Check sheet for the drawn part. Datum: minimum x, y, z corner. Units: mm. Round coordinates to 2 decimals unless told otherwise and drop trailing zeros. Write each loop counter-clockwise with the first axis right and the second up, starting at its lowest first coordinate (ties: lowest second). Pieces come first, ordered by that corner, then holes. Notation, with made-up numbers: M 63.5,24 L 75.5,24 A21 ccw 75.5,48 Z; hole C 58.25,89.25 d11. An arc over 180 degrees is marked long. One line per item, written item: value. Start each with the question number.
1. Section check B-B (y = 4.75). Record the boundary of the cut face in (x, z).
2. Section check A-A (z = 17.5). Record the boundary of the cut face in (x, y), and give its area (3 significant figures).
3. Release check for a two-part mould opening along X. For the marked faces 1, 2 and 3 record: pulls with the +X half, pulls with the -X half, needs draft (parallel to the pull), parting line crosses it, or undercut.
4. Depth check by flat-ended pin: P1, Ø1.5, axis at x = 13.5, y = 7.5, coming from the -Z side; P2, Ø3, axis at y = 12, z = 24.5, coming from the -X side; P3, Ø8, axis at y = 2, z = 10.5, coming from the -X side. Enter the tip coordinate at first touch or a pass-through.
5. Scan lines: probe 1 along Z at (x, y) = (17.5, 11); probe 2 along Z at (x, y) = (18, 6.5); probe 3 along Z at (x, y) = (10.5, 8.5). Record each from-to range of solid material in increasing order. Write a range as [from, to].
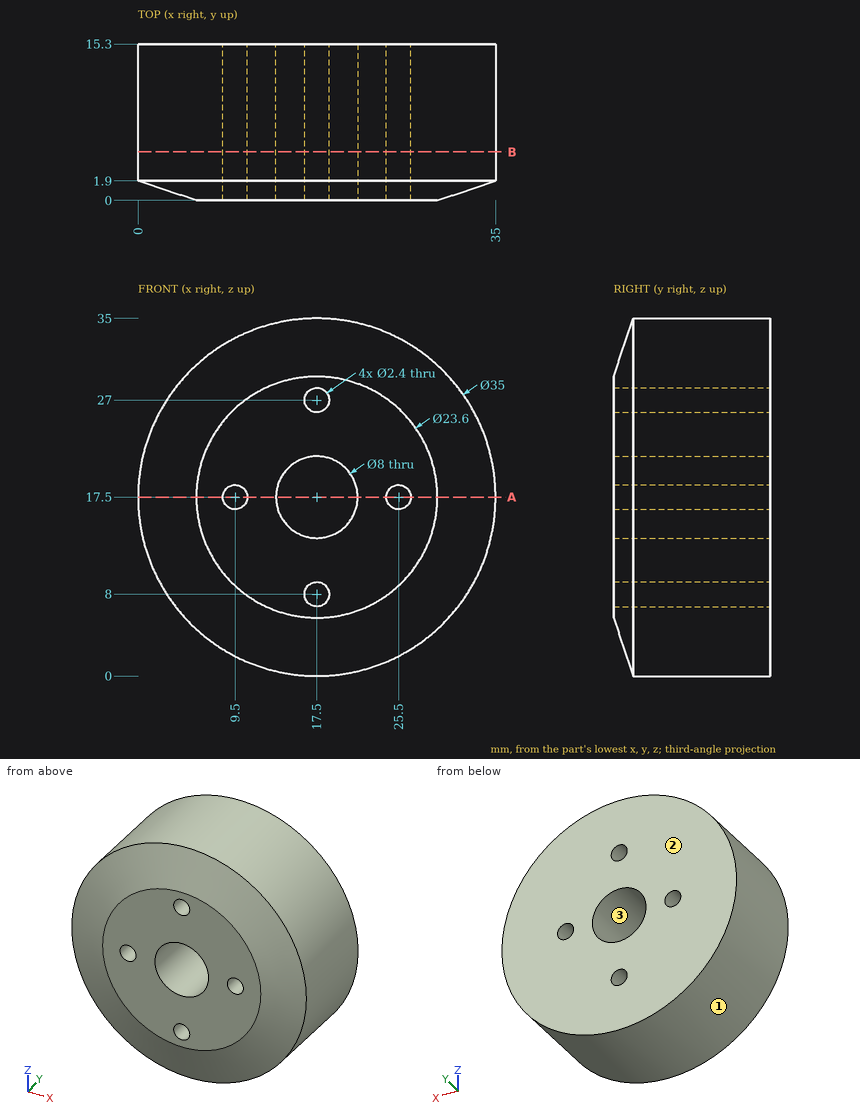
Result sheet:
1. outline: C 17.5,17.5 d35; hole C 9.5,17.5 d2.4; hole C 17.5,17.5 d8; hole C 17.5,8 d2.4; hole C 17.5,27 d2.4; hole C 25.5,17.5 d2.4
2. outline: M 0,1.9 L 5.7,0 L 8.3,0 L 8.3,15.3 L 0,15.3 Z; M 10.7,0 L 13.5,0 L 13.5,15.3 L 10.7,15.3 Z; M 21.5,0 L 24.3,0 L 24.3,15.3 L 21.5,15.3 Z; M 26.7,0 L 29.3,0 L 35,1.9 L 35,15.3 L 26.7,15.3 Z
2. area: 329 mm2
3. face 1: parting line crosses it
3. face 2: needs draft
3. face 3: undercut
4. P1: stops at z = 0.3
4. P2: stops at x = 0.89
4. P3: stops at x = 0.26
5. probe 1: z = [0, 6.8], [9.2, 13.5], [21.5, 25.8], [28.2, 35]
5. probe 2: z = [0.01, 6.91], [9.09, 13.53], [21.47, 25.91], [28.09, 34.99]
5. probe 3: z = [1.46, 16.84], [18.16, 33.54]
